```python
from build123d import *

# Parameters (mm, degrees)
F0_W     = 8
F0_H     = 30
F1_DEPTH = 25
F5_DEPTH = 2.25
F7_DEPTH = 2.251


# Not quite as in the source:
# - a feature of the source that left no trace in its solid (it failed there, or was rolled back) is left out


with BuildPart() as f1:
    # F0 (on Top) → F1 (new body)
    with BuildSketch(Plane.XY):
        with Locations((4.3632484525, -0.778583717)):
            Rectangle(F0_W, F0_H)
    extrude(amount=F1_DEPTH)

    # F4 (on offset) → F5 (cut, through all)
    with BuildSketch(Plane.YZ.offset(3.8632484525)):
        with BuildLine():
            Line((-10, 26.291980999), (-10, 12))
            ThreePointArc((-10, 12), (0, 2), (10, 12))
            Line((10, 12), (10, 26.291980999))
            Line((10, 26.291980999), (-10, 26.291980999))
        make_face()
    extrude(amount=F5_DEPTH, mode=Mode.SUBTRACT)

    # F6 (on offset) → F7 (cut, through all)
    with BuildSketch(Plane.YZ.offset(6.1132484525)):
        with BuildLine():
            Line((-5, 26.8745111924), (-5, 12))
            ThreePointArc((-5, 12), (0, 7), (5, 12))
            Line((5, 12), (5, 26.8745111924))
            Line((5, 26.8745111924), (-5, 26.8745111924))
        make_face()
    extrude(amount=F7_DEPTH, mode=Mode.SUBTRACT)


solid = f1.part
```
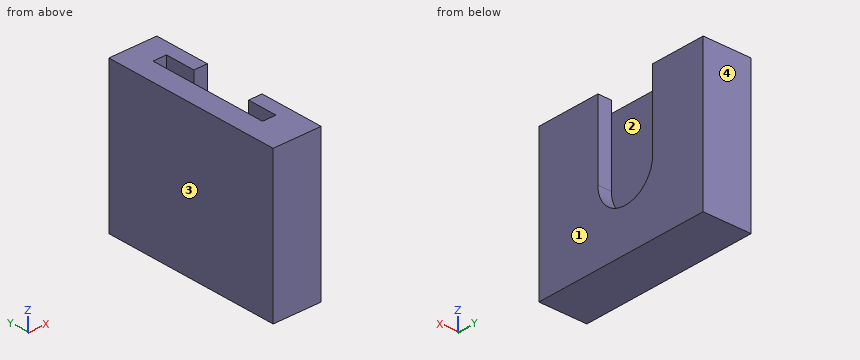
Work out the finished part from the listing and answer in its coordinate system (mm). Face numbers are marked on the shaded views. Give positions to 0.01 mm unless a question says otherwise; leave off trailing zeros. Write each loop counter-clockwise with the first axis right and the second up, starting at its lowest first coordinate (ties: lowest second). Pieces come first, ordered by that corner, then holes.
(1) The mould has two halves that part along X. Classify the marked faces 1, 2, 3 and 4: pulls with the +X half, pulls with the -X half, needs draft (parallel to the pull), parting line crosses it, or undercut.
Final values:
face 1: pulls with the +X half
face 2: undercut
face 3: pulls with the -X half
face 4: needs draft
(2) The part is cut by section B-B on z = 17. Write down the section's boundary in (x, y), plus the area to 4 significant figures.
Final values:
outline: (0.36, -15.78) - (8.36, -15.78) - (8.36, -5) - (6.11, -5) - (6.11, -10) - (3.86, -10) - (3.86, 10) - (6.11, 10) - (6.11, 5) - (8.36, 5) - (8.36, 14.22) - (0.36, 14.22) - close
area: 172.5 mm2
(3) The part is cut by section A-A on x = 7. Write down the section's boundary in (y, z), plus the area to 3 significant figures.
Final values:
outline: (-15.78, 0) - (14.22, 0) - (14.22, 25) - (5, 25) - (5, 12) arc R5 cw to (-5, 12) - (-5, 25) - (-15.78, 25) - close
area: 581 mm2
(4) Flat-ended cylindrical pins translate along their axes: pin 1 Ø1.5 at (y, z) = (0.5, 21) entering from +X; pin 2 Ø1 at (y, z) = (-2, 7.5) entering from +X. Find the tip coordinate at first contact, or state that the pin passes through.
Final values:
pin 1: stops at x = 3.86
pin 2: stops at x = 8.36
(5) The part is cut by section C-C on y = 0. Write down the section's boundary in (x, z).
Final values:
outline: (0.36, 0) - (8.36, 0) - (8.36, 7) - (6.11, 7) - (6.11, 2) - (3.86, 2) - (3.86, 25) - (0.36, 25) - close
(6) Straight lines are drawn through the part: line 1 (Y direction, x = 7.75, z = 11.75); line 2 (X direction, y = -9.25, z = 8.5); line 3 (Y direction, x = 5.5, z = 14.5). For each, find the intervals that lie inside material, in ascending order.
Final values:
line 1: y = -15.78 to -4.99, 4.99 to 14.22
line 2: x = 0.36 to 3.86, 6.11 to 8.36
line 3: y = -15.78 to -10, 10 to 14.22
(7) The part is cut by section D-D on z = 3.75. Write down the section's boundary in (x, y), plus the area to 3 significant figures.
Final values:
outline: (0.36, -15.78) - (8.36, -15.78) - (8.36, 14.22) - (0.36, 14.22) - close; hole (3.86, -5.65) - (6.11, -5.65) - (6.11, 5.65) - (3.86, 5.65) - close
area: 215 mm2
